Geometry: final body of the model. Coordinates: model frame, mm. Face numbers are marked on the shaded views. A direction names the side the tool comes from. Give positions to 0.01 mm unless a question says otherwise; leave off trailing zeros. Order: outer loops, then holes, each group sorted by start corner. A loop starts at its lowest first (then second) coordinate and runs counter-clockwise, first axis right, second up. Notation, with made-up numbers: (30.5, 38.5) - (41.5, 38.5) arc R17 ccw to (41.5, 70.5) - close; hole circle Ø8 at (1, -21). An arc over 180 degrees is marked (long way). One line per item, written item: value.
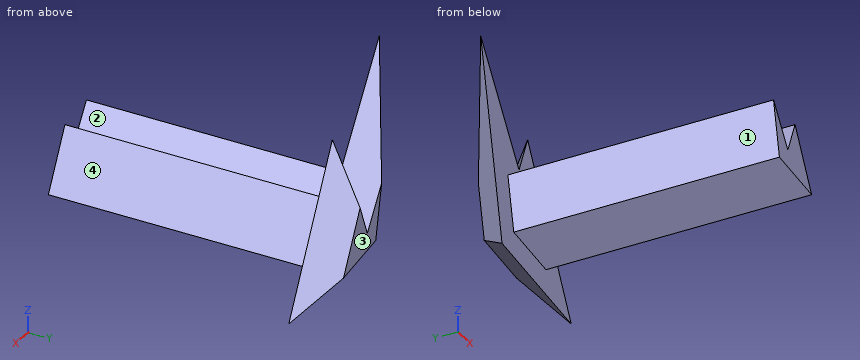
```python
from build123d import *

# Parameters (mm, degrees)
F1_DEPTH = 150
F2_DEPTH = 15
F2_TAPER = -40


with BuildPart() as f1:
    # F0 (on Front) → F1 (new body)
    with BuildSketch(Plane.XZ):
        Polygon((-1.5002588741, -3.1941000372), (-14.446044527, 15.9221046604), (-9.1225432232, -10.6953958049), (20.0357193127, -15.1719756424), (5.0331273116, 13.1393668242), align=None)
    extrude(amount=F1_DEPTH)

    # F0 (on Front) → F2 (join)
    with BuildSketch(Plane.XZ):
        Polygon((-1.5002588741, -3.1941000372), (-14.446044527, 15.9221046604), (-9.1225432232, -10.6953958049), (20.0357193127, -15.1719756424), (5.0331273116, 13.1393668242), align=None)
    extrude(amount=F2_DEPTH, taper=F2_TAPER)


solid = f1.part
```
1) First-contact query: pin 1 (5 mm diameter, centred on x = 14, y = -85, fed in from -Z); pin 2 (1.5 mm diameter, centred on y = -32.5, z = 6.5, fed in from -X); pin 3 (10 mm diameter, centred on x = 0.5, z = 31, fed in from -Y). Flat tips, straight axial feed; report the tip coordinate or a pass-through.
Answers below:
pin 1: z = -14.63
pin 2: x = -12.71
pin 3: y = -15
2) Material intervals for line 1 along X through (y, z) = (-6, 21); line 2 along X through (y, z) = (-72.5, 6.5); line 3 along Z through (x, y) = (-8.5, -119), sorted ascending.
Answers below:
line 1: -20.6 to -11.8, 2.75 to 6.57
line 2: -12.56 to -8.07, 2.38 to 8.55
line 3: -10.79 to 7.14
3) Set-up query: the marked faces 1, 2, 3 and 4. Return all of +Z, -Z, +X, -X, +Y, -Y with unobstructed straight access to the full face (end or side cutting, diameter ignored); none if empty.
Answers below:
face 1: -Z, -X, -Y
face 2: +Z, -Y
face 3: +Z, -Z, +X, -X, +Y
face 4: +Z, +X, -Y
4) Section A-A, the plane y = -66.5. Return loops of the section in (x, z), then the cut area to 3 significant figures.
Answers below:
outline: (-14.45, 15.92) - (-9.12, -10.7) - (20.04, -15.17) - (5.03, 13.14) - (-1.5, -3.19) - close
area: 463 mm^2
